Verification items for the finished model (mm, model axes). Round coordinates to 2 decimals unless told otherwise and drop trailing zeros. Write each loop counter-clockwise with the first axis right and the second up, starting at its lowest first coordinate (ties: lowest second). Pieces come first, ordered by that corner, then holes.
from build123d import *
from build123d.topology import SkipClean

# Parameters (mm, degrees)
ESQUISSE1_R        = 5
BOSS_EXTRU_1_DEPTH = 3


with BuildPart() as part:
    # Esquisse1 → Boss.-Extru.1 (new body)
    with BuildSketch(Plane.XY):
        with BuildLine():
            Line((45, 39), (45, 60))
            Line((45, 60), (-20, 60))
            Line((-20, 60), (-20, 0))
            Line((-20, 0), (45, 0))
            Line((45, 0), (45, 29))
            ThreePointArc((45, 29), (40, 34), (45, 39))
        make_face()
        with Locations((-10, 50)):
            Circle(ESQUISSE1_R, mode=Mode.SUBTRACT)
        with Locations((-10, 10)):
            Circle(ESQUISSE1_R, mode=Mode.SUBTRACT)
    boss_extru_1 = extrude(amount=BOSS_EXTRU_1_DEPTH)

    # Symétrie1: Boss.-Extru.1 across plane
    with SkipClean():  # the faces are left unmerged after this step: merging them gives an invalid solid
        add(boss_extru_1.mirror(Plane(origin=(45, 0, 3), x_dir=(0, 0, 1), z_dir=(1, 0, 0))))


solid = part.part
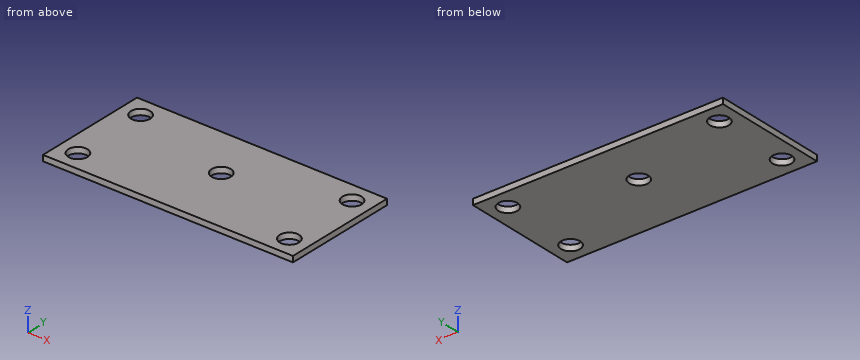
Q1. Depth check by flat-ended pin: P1, Ø16, axis at x = 100, y = 50, coming from the -Z side; P2, Ø9, axis at x = 45, y = 34, coming from the +Z side. Enter the tip coordinate at first touch or a pass-through.
Recorded:
P1: stops at z = 0
P2: passes through
Q2. Sectioned sample at B-B (x = 100). Enter the section's corners in (y, z).
Recorded:
outline: (0, 0) - (5, 0) - (5, 3) - (0, 3) - close; (15, 0) - (45, 0) - (45, 3) - (15, 3) - close; (55, 0) - (60, 0) - (60, 3) - (55, 3) - close
Q3. Sectioned sample at C-C (y = 10). Enter the section's corners in (x, z).
Recorded:
outline: (-20, 0) - (-15, 0) - (-15, 3) - (-20, 3) - close; (-5, 0) - (95, 0) - (95, 3) - (-5, 3) - close; (105, 0) - (110, 0) - (110, 3) - (105, 3) - close
Q4. Material ranges on line 1 along Y through (x, z) = (100, 2.25); line 2 along Y through (x, z) = (45, 1.9); line 3 along X through (y, z) = (33.5, 1.5), recorded low to high.
Recorded:
line 1: y = 0 to 5, 15 to 45, 55 to 60
line 2: y = 0 to 29, 39 to 60
line 3: x = -20 to 40.03, 49.97 to 110
Q5. Sectioned sample at A-A (y = 34). Enter the section's corners in (x, z).
Recorded:
outline: (-20, 0) - (40, 0) - (40, 3) - (-20, 3) - close; (50, 0) - (110, 0) - (110, 3) - (50, 3) - close
Q6. Sectioned sample at D-D (z = 1.55). Enter the section's corners in (x, y), plus the area to 3 significant figures.
Recorded:
outline: (-20, 0) - (110, 0) - (110, 60) - (-20, 60) - close; hole circle Ø10 at (-10, 10); hole circle Ø10 at (-10, 50); hole circle Ø10 at (45, 34); hole circle Ø10 at (100, 10); hole circle Ø10 at (100, 50)
area: 7,410 mm2
